Check sheet for the modelled part. Datum: model origin and axes. Units: mm. A direction names the side the tool comes from. Give positions to 0.01 mm unless a question says otherwise; leave off trailing zeros. Order: outer loops, then holes, each group sorted by start corner. A loop starts at its lowest first (then second) coordinate and runs counter-clockwise, first axis right, second up. Notation, with made-up numbers: M -35.5,-2 L -3.5,-2 A31 cw -3.5,37 Z; hole C -4.5,-21.5 d10. An arc over 180 degrees is marked long. Return JSON: item names as keys, results as strings. Group by question number.
from build123d import *

# Parameters (mm, degrees)
BOSS_EXTRUDE1_DEPTH = 20
SKETCH3_R           = 3.15
CUT_EXTRUDE1_DEPTH  = 42.243181255
SKETCH5_R           = 2.25
CUT_EXTRUDE2_DEPTH  = 40.420806689
FILLET1_R           = 1


with BuildPart() as part:
    # Sketch2 → Boss-Extrude1 (new body)
    with BuildSketch(Plane.XY):
        Polygon((-12, 0), (12, 0), (12, -23), (25, -23), (25, -20), (15, -20), (15, 3), (-15, 3), (-15, -20), (-25, -20), (-25, -23), (-12, -23), align=None)
    extrude(amount=BOSS_EXTRUDE1_DEPTH)

    # Sketch3 → Cut-Extrude1 (cut, through all)
    with BuildSketch(Plane(origin=(0, 3, 0), x_dir=(1, 0, 0), z_dir=(0, 1, 0))):
        with Locations(Location((4, -10, 0), (0, 0, 180))):
            Circle(SKETCH3_R)
    extrude(amount=-CUT_EXTRUDE1_DEPTH, mode=Mode.SUBTRACT)

    # Sketch5 → Cut-Extrude2 (cut, through all)
    with BuildSketch(Plane(origin=(0, -20, 0), x_dir=(1, 0, 0), z_dir=(0, 1, 0))):
        with Locations(Location((-20, -10, 0), (0, 0, 180))):
            Circle(SKETCH5_R)
        with Locations(Location((20, -10, 0), (0, 0, 180))):
            Circle(SKETCH5_R)
    extrude(amount=-CUT_EXTRUDE2_DEPTH, mode=Mode.SUBTRACT)

    # Fillet1
    fillet1_edges = [part.edges().sort_by_distance(p)[0] for p in [
        (15, -20, 10),
        (25, -20, 10),
        (25, -23, 10),
        (12, -23, 10),
        (12, 0, 10),
        (-12, 0, 10),
        (-12, -23, 10),
        (-25, -23, 10),
        (-25, -20, 10),
        (-15, -20, 10),
        (-15, 3, 10),
        (15, 3, 10),
    ]]
    fillet(fillet1_edges, radius=FILLET1_R)


solid = part.part
1) Sectioned sample at A-A on y = -5.25. Record the boundary of the cut face in (x, z), then the cut area to 3 significant figures.
2) Tool access check on faces 1 (the face through (-11.699, -0.285, 10.14)), 2 (the face through (-19.9, -20, 7.6)), 3 (the face through (15, -9, 10)). Record the directions out of +Z, -Z, +X, -X, +Y, -Y that give a thin tool (end or side, any length) a straight path to the whole face; none if there is none.
3) Material ranges on line 1 along Z through (x, y) = (20, -22.05); line 2 along Z through (x, y) = (4, 2.15); line 3 along X through (y, z) = (-10, 1.25), recorded low to high.
4) Sectioned sample at B-B on x = 20. Record the boundary of the cut face in (y, z), then the cut area to 3 significant figures.
5) Sectioned sample at D-D on z = 5. Record the boundary of the cut face in (x, y), then the cut area to 3 significant figures.
6) Sectioned sample at C-C on y = 1. Record the boundary of the cut face in (x, z), then the cut area to 3 significant figures.
7) Depth check by flat-ended pin: P1, Ø3, axis at x = 17.5, z = 16.5, coming from the +Y side; P2, Ø6, axis at y = -5, z = 9.5, coming from the +X side; P3, Ø3.5, axis at x = -20, z = 10, coming from the +Y side; P4, Ø6, axis at y = -16, z = 7, coming from the -X side. Enter the tip coordinate at first touch or a pass-through.
8) Release check for a two-part mould opening along Z. For faces 4 (the face through (4.41, 1.521, 13.123)), 5 (the face through (24.715, -20.301, 10.14)) record: released by +Z, released by -Z, zero draft, split by the parting line, or undercut.
Reply:
{
 "1": {"outline": "M -15,0 L -12,0 L -12,20 L -15,20 Z; M 12,0 L 15,0 L 15,20 L 12,20 Z", "area": "120 mm^2"},
 "2": {"face 1": "+Z, -Z, -Y", "face 2": "+Z, -Z, -X, +Y", "face 3": "+Z, -Z, +X, +Y"},
 "3": {"line 1": "0 to 7.75, 12.25 to 20", "line 2": "0 to 6.85, 13.15 to 20", "line 3": "-15 to -12, 12 to 15"},
 "4": {"outline": "M -23,0 L -20,0 L -20,7.75 L -23,7.75 Z; M -23,12.25 L -20,12.25 L -20,20 L -23,20 Z", "area": "46.5 mm^2"},
 "5": {"outline": "M -25,-22 A1 ccw -24,-23 L -13,-23 A1 ccw -12,-22 L -12,-1 A1 cw -11,0 L 11,0 A1 cw 12,-1 L 12,-22 A1 ccw 13,-23 L 24,-23 A1 ccw 25,-22 L 25,-21 A1 ccw 24,-20 L 16,-20 A1 cw 15,-19 L 15,2 A1 ccw 14,3 L -14,3 A1 ccw -15,2 L -15,-19 A1 cw -16,-20 L -24,-20 A1 ccw -25,-21 Z", "area": "287 mm^2"},
 "6": {"outline": "M -15,0 L 15,0 L 15,20 L -15,20 Z; hole C 4,10 d6.3", "area": "569 mm^2"},
 "7": {"P1": "y = -20", "P2": "x = 15", "P3": "through", "P4": "x = -15"},
 "8": {"face 4": "undercut", "face 5": "zero draft"}
}
